```python
from build123d import *

# Parameters (mm, degrees)
IZIM1_W                     = 40.5
IZIM1_H                     = 18
Y_KSEKLIK_EKSTR_ZYON1_DEPTH = 1.5
IZIM2_R                     = 1.1
KES_EKSTR_ZYON1_DEPTH       = 1.5
IZIM3_W                     = 6
IZIM3_H                     = 6
Y_KSEKLIK_EKSTR_ZYON2_DEPTH = 4.8
IZIM4_W                     = 6
IZIM4_H                     = 9
Y_KSEKLIK_EKSTR_ZYON3_DEPTH = 3
KES_EKSTR_ZYON2_DEPTH       = 6
KES_EKSTR_ZYON3_DEPTH       = 5
IZIM8_R                     = 0.5
KES_EKSTR_ZYON4_DEPTH       = 5
Y_KSEKLIK_EKSTR_ZYON4_START = 4
Y_KSEKLIK_EKSTR_ZYON4_DEPTH = 4


with BuildPart() as part:
    # izim1 → Y_kseklik-Ekstr_zyon1 (new body)
    with BuildSketch(Plane.XY):
        Rectangle(IZIM1_W, IZIM1_H)
    extrude(amount=Y_KSEKLIK_EKSTR_ZYON1_DEPTH)

    # izim2 → Kes-Ekstr_zyon1 (cut)
    with BuildSketch(Plane(origin=(0, 0, 0), x_dir=(-1, 0, 0), z_dir=(0, 0, -1))):
        with Locations((-18.75, 7.5)):
            Circle(IZIM2_R)
        with Locations(Location((-18.75, -7.5, 0), (0, 0, 180))):
            Circle(IZIM2_R)
    extrude(amount=-KES_EKSTR_ZYON1_DEPTH, mode=Mode.SUBTRACT)

    # izim3 → Y_kseklik-Ekstr_zyon2 (add)
    with BuildSketch(Plane(origin=(0, 0, 0), x_dir=(-1, 0, 0), z_dir=(0, 0, -1))):
        with Locations((5.25, 5.7)):
            Rectangle(IZIM3_W, IZIM3_H)
    extrude(amount=Y_KSEKLIK_EKSTR_ZYON2_DEPTH)

    # izim4 → Y_kseklik-Ekstr_zyon3 (add)
    with BuildSketch(Plane(origin=(0, 0, 0), x_dir=(-1, 0, 0), z_dir=(0, 0, -1))):
        with Locations((15.25, 0)):
            Rectangle(IZIM4_W, IZIM4_H)
    extrude(amount=Y_KSEKLIK_EKSTR_ZYON3_DEPTH)

    # izim6 → Kes-Ekstr_zyon2 (cut)
    with BuildSketch(Plane.ZY.offset(18.25)):
        with BuildLine():
            ThreePointArc((-2.960618191, -4.326328271), (-2.980432326, -4.320748503), (-3, -4.314357896))
            Line((-3, -4.314357896), (-3, -4.5))
            Line((-3, -4.5), (-1.6, -4.5))
            ThreePointArc((-1.6, -4.5), (-2.285828647, -4.456406648), (-2.960618191, -4.326328271))
        make_face()
        with BuildLine():
            ThreePointArc((-0.239381809, -4.326328271), (-0.914171353, -4.456406648), (-1.6, -4.5))
            Line((-1.6, -4.5), (0, -4.5))
            Line((0, -4.5), (0, -4.184107288))
            ThreePointArc((0, -4.184107288), (-0.109591088, -4.272217467), (-0.239381809, -4.326328271))
        make_face()
        with BuildLine():
            Line((0, 4.5), (-1.60000002, 4.5))
            ThreePointArc((-1.60000002, 4.5), (-0.914171363, 4.456406649), (-0.239381809, 4.326328271))
            ThreePointArc((-0.239381809, 4.326328271), (-0.109591088, 4.272217467), (0, 4.184107288))
            Line((0, 4.184107288), (0, 4.5))
        make_face()
        with BuildLine():
            Line((-3, 4.5), (-3, 4.314357896))
            ThreePointArc((-3, 4.314357896), (-2.980432326, 4.320748503), (-2.960618191, 4.326328271))
            ThreePointArc((-2.960618191, 4.326328271), (-2.285828657, 4.456406647), (-1.60000002, 4.5))
            Line((-1.60000002, 4.5), (-3, 4.5))
        make_face()
    extrude(amount=-KES_EKSTR_ZYON2_DEPTH, mode=Mode.SUBTRACT)

    # izim7 → Kes-Ekstr_zyon3 (cut)
    with BuildSketch(Plane.ZY.offset(18.25)):
        with BuildLine():
            Line((-0.3, -4.031510098), (-0.3, 4.031510098))
            ThreePointArc((-0.3, 4.031510098), (-0.307326862, 4.033870403), (-0.314739124, 4.035947013))
            ThreePointArc((-0.314739124, 4.035947013), (-1.504744914, 4.199113259), (-2.7, 4.080360227))
            Line((-2.7, 4.080360227), (-2.7, -4.080360227))
            ThreePointArc((-2.7, -4.080360227), (-1.504744914, -4.199113259), (-0.314739124, -4.035947013))
            ThreePointArc((-0.314739124, -4.035947013), (-0.307326862, -4.033870403), (-0.3, -4.031510098))
        make_face()
    extrude(amount=-KES_EKSTR_ZYON3_DEPTH, mode=Mode.SUBTRACT)

    # izim8 → Kes-Ekstr_zyon4 (cut)
    with BuildSketch(Plane(origin=(0, 0, 0), x_dir=(-1, 0, 0), z_dir=(0, 0, -1))):
        with Locations((15.25, 8.2)):
            Circle(IZIM8_R)
        with Locations((15.25, -8.2)):
            Circle(IZIM8_R)
    extrude(amount=-KES_EKSTR_ZYON4_DEPTH, mode=Mode.SUBTRACT)

    # izim9 → Y_kseklik-Ekstr_zyon4 (add)
    with BuildSketch(Plane.ZY.offset(18.25).offset(Y_KSEKLIK_EKSTR_ZYON4_START)):
        with BuildLine():
            ThreePointArc((-2.960618191, -4.326328271), (-1.6, -4.5), (-0.239381809, -4.326328271))
            ThreePointArc((-0.239381809, -4.326328271), (-0.109591088, -4.272217467), (0, -4.184107288))
            Line((0, -4.184107288), (0, 4.184107288))
            ThreePointArc((0, 4.184107288), (-0.109591088, 4.272217467), (-0.239381809, 4.326328271))
            ThreePointArc((-0.239381809, 4.326328271), (-1.6, 4.5), (-2.960618191, 4.326328271))
            ThreePointArc((-2.960618191, 4.326328271), (-2.980432326, 4.320748503), (-3, 4.314357896))
            Line((-3, 4.314357896), (-3, -4.314357896))
            ThreePointArc((-3, -4.314357896), (-2.980432326, -4.320748503), (-2.960618191, -4.326328271))
        make_face()
        with BuildLine():
            ThreePointArc((-0.314739124, -4.035947013), (-1.504744914, -4.199113259), (-2.7, -4.080360227))
            Line((-2.7, -4.080360227), (-2.7, 4.080360227))
            ThreePointArc((-2.7, 4.080360227), (-1.504744914, 4.199113259), (-0.314739124, 4.035947013))
            ThreePointArc((-0.314739124, 4.035947013), (-0.307326862, 4.033870403), (-0.3, 4.031510098))
            Line((-0.3, 4.031510098), (-0.3, -4.031510098))
            ThreePointArc((-0.3, -4.031510098), (-0.307326862, -4.033870403), (-0.314739124, -4.035947013))
        make_face(mode=Mode.SUBTRACT)
    extrude(amount=-Y_KSEKLIK_EKSTR_ZYON4_DEPTH)


solid = part.part
```
CAD build for the part. Positions are in the model's coordinates, mm. A direction names the side the tool comes from. Round coordinates to 2 decimals unless told otherwise and drop trailing zeros. Loops run counter-clockwise (first coordinate to the right, second up) from the corner with the lowest first, then second, coordinate; pieces in that order, holes last. Notation, with made-up numbers: M 43.25,-23.75 L 63.25,-23.75 A34 ccw 63.25,9.25 Z; hole C 8.25,-10 d4. An arc over 180 degrees is marked long. Return JSON: item names as keys, results as strings. Group by question number.
(1) Saw through at B-B, the plane y = -8.2. List the corners of the cut face in (x, z), and give its area (3 significant figures).
(2) Mould opens along Z. For faces 1 (the flat face through (-21, 0, 0)), 2 (the flat face through (-12.25, 0, -1)), 3 (the flat face through (-18, 0, -2.7)), 4 (the cylindrical face through (-17.8, 4.2, -1.5)) say: +Z half, -Z half, draft (parallel to the pull), parting line (faces both ways), or undercut.
(3) Wall check: probe 1 along Y at (x, z) = (18.75, 0.45); probe 2 along X at (y, z) = (-7.5, 0.8); probe 3 along X at (y, z) = (3.75, -0.75). Give the ranges that are in metal, low to high. Write a range as [from, to].
(4) Drop flat-ended pins along their axis: P1, Ø5.5, axis at x = 2, y = 2.5, coming from the -Z side; P2, Ø2.5, axis at x = -5, z = -1.5, coming from the +Y side; P3, Ø4.5, axis at x = -16, y = -1, coming from the -Z side. Give the stop position or say it passes through.
(5) Tool access for faces 5 (the flat face through (-5, 8.7, -2)), 6 (the flat face through (-5, 2.7, -2)), 7 (the flat face through (-20.25, 0, 1)): list every direction of +Z, -Z, +X, -X, +Y, -Y with a clear straight run to the whole face (end or side of a thin tool).
(6) Saw through at A-A, the plane x = 18.75. List the corners of the cut face in (y, z), and give its area (3 significant figures).
(7) Saw through at C-C, the plane z = -0.75. List the corners of the cut face in (x, y), and give its area (3 significant figures).
Answer list:
{
 "1": {"outline": "M -20.25,0 L -15.75,0 L -15.75,1.5 L -20.25,1.5 Z; M -14.75,0 L 17.9,0 L 17.9,1.5 L -14.75,1.5 Z; M 19.6,0 L 20.25,0 L 20.25,1.5 L 19.6,1.5 Z", "area": "56.7 mm2"},
 "2": {"face 1": "+Z half", "face 2": "draft", "face 3": "undercut", "face 4": "undercut"},
 "3": {"probe 1": "[-9, -8.6], [-6.4, 6.4], [8.6, 9]", "probe 2": "[-20.25, 17.65], [19.85, 20.25]", "probe 3": "[-13.25, -12.25], [-8.25, -2.25]"},
 "4": {"P1": "z = 0", "P2": "y = 8.7", "P3": "z = -3"},
 "5": {"face 5": "-Z, +X, -X, +Y", "face 6": "-Z, +X, -Y", "face 7": "+Z, -X, +Y, -Y"},
 "6": {"outline": "M -9,0 L -8.6,0 L -8.6,1.5 L -9,1.5 Z; M -6.4,0 L 6.4,0 L 6.4,1.5 L -6.4,1.5 Z; M 8.6,0 L 9,0 L 9,1.5 L 8.6,1.5 Z", "area": "20.4 mm2"},
 "7": {"outline": "M -22.25,-4.43 L -12.25,-4.43 L -12.25,4.43 L -22.25,4.43 L -22.25,4.13 L -13.25,4.13 L -13.25,-4.13 L -22.25,-4.13 Z; M -8.25,2.7 L -2.25,2.7 L -2.25,8.7 L -8.25,8.7 Z", "area": "50.3 mm2"}
}
